from build123d import *

# Parameters (mm, degrees)
BOSS_EXTRUDE1_DEPTH = 4
SKETCH2_R           = 3.1
CUT_EXTRUDE2_DEPTH  = 4
SKETCH3_R           = 1.25
BOSS_EXTRUDE2_DEPTH = 4


with BuildPart() as part:
    # Sketch1 → Boss-Extrude1 (new body)
    with BuildSketch(Plane(origin=(0, 23.1, 0), x_dir=(1, 0, 0), z_dir=(0, 1, 0))):
        with BuildLine():
            Line((5.5, 6.5), (-21.3, 6.5))
            Line((-21.3, 6.5), (-21.3, -6.5))
            Line((-21.3, -6.5), (5.5, -6.5))
            ThreePointArc((5.5, -6.5), (12, 0), (5.5, 6.5))
        make_face()
    extrude(amount=BOSS_EXTRUDE1_DEPTH)

    # Sketch2 → Cut-Extrude2 (cut)
    with BuildSketch(Plane(origin=(0, 23.1, 0), x_dir=(1, 0, 0), z_dir=(0, 1, 0))):
        with Locations(Location((5.5, 0, 0), (0, 0, 270))):
            Circle(SKETCH2_R)
    extrude(amount=CUT_EXTRUDE2_DEPTH, mode=Mode.SUBTRACT)

    # Sketch3 → Boss-Extrude2 (add)
    with BuildSketch(Plane(origin=(0, 19.1, 0), x_dir=(1, 0, 0), z_dir=(0, 1, 0))):
        with Locations(Location((-18.8, -4.5, 0), (0, 0, 270))):
            Circle(SKETCH3_R)
        with Locations(Location((-18.8, 4.5, 0), (0, 0, 270))):
            Circle(SKETCH3_R)
    extrude(amount=BOSS_EXTRUDE2_DEPTH)


solid = part.part
Design review of the part built by this model. Coordinates are the model's own, in mm. A direction names the side the tool comes from. Round coordinates to 2 decimals unless told otherwise and drop trailing zeros. Order: outer loops, then holes, each group sorted by start corner. A loop starts at its lowest first (then second) coordinate and runs counter-clockwise, first axis right, second up.
1) Draft analysis for pull direction X (two halves, no side actions). For faces 1 (the flat face through (-21.3, 25, 0)), 2 (the cylindrical face through (2.474, 25.072, -0.672)), 3 (the flat face through (-8, 25, 6.5)), 4 (the cylindrical face through (-17.746, 21.072, 5.172)), state which applies: released by +X, released by -X, zero draft, split by the parting line, or undercut.
The answers:
face 1: released by -X
face 2: undercut
face 3: zero draft
face 4: split by the parting line
2) For L1, parallel to X at y = 24.45, z = 0; L2, parallel to Y at x = -17.5, z = 1; L3, parallel to X at y = 25.25, z = -2.75, list the stretches that pass through material, from the lowest coordinate up.
The answers:
L1: x = -21.3 to 2.4, 8.6 to 12
L2: y = 23.1 to 27.1
L3: x = -21.3 to 4.07, 6.93 to 11.39
3) Clearance check with flat-ended pins moving along their axes: pin 1 Ø6 at (x, z) = (7, 0.5) entering from -Y; pin 2 Ø1.5 at (y, z) = (22, 4.5) entering from -X; pin 3 Ø1 at (y, z) = (23, -3.5) entering from +X. State where each tip first meets the part, or that it passes through.
The answers:
pin 1: stops at y = 23.1
pin 2: stops at x = -20.05
pin 3: stops at x = 11.26
4) Consider section C-C (y = 22.5). State the section outline as (x, z) points.
The answers:
outline: circle Ø2.5 at (-18.8, -4.5); circle Ø2.5 at (-18.8, 4.5)
5) Consider section A-A (z = 0). State the section outline as (x, y) points.
The answers:
outline: (-21.3, 23.1) - (2.4, 23.1) - (2.4, 27.1) - (-21.3, 27.1) - close; (8.6, 23.1) - (12, 23.1) - (12, 27.1) - (8.6, 27.1) - close
6) Consider section B-B (y = 25.25). State the section outline as (x, z) points.
The answers:
outline: (-21.3, -6.5) - (5.5, -6.5) arc R6.5 ccw to (5.5, 6.5) - (-21.3, 6.5) - close; hole circle Ø6.2 at (5.5, 0)
7) Machinability: for faces 5 (the cylindrical face through (-17.56, 21.07, -4.66)), 6 (the flat face through (-5, 27.1, 0)), which of the approach directions +Z, -Z, +X, -X, +Y, -Y give a long, thin tool a straight path to every point of the face, cutting with its end or side? Answer none if there is none.
The answers:
face 5: -Y
face 6: +Z, -Z, +X, -X, +Y
8) Consider section D-D (z = -2.25). State the section outline as (x, y) points, plus the area to 3 significant figures.
The answers:
outline: (-21.3, 23.1) - (3.37, 23.1) - (3.37, 27.1) - (-21.3, 27.1) - close; (7.63, 23.1) - (11.6, 23.1) - (11.6, 27.1) - (7.63, 27.1) - close
area: 115 mm2
